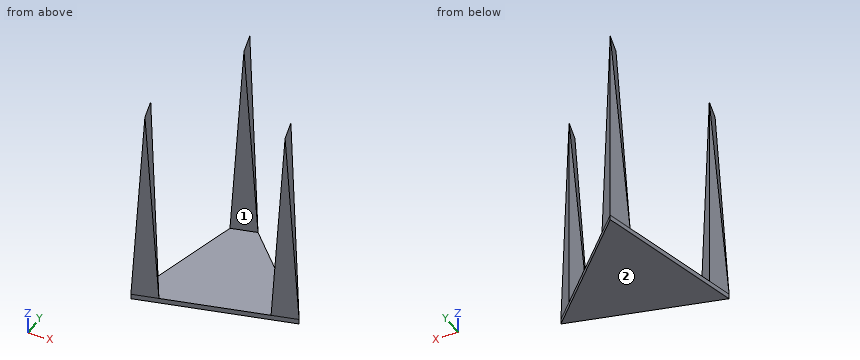
```python
from build123d import *

# Parameters (mm, degrees)
F1_DEPTH = 1
F3_DEPTH = 40
F5_DEPTH = 4.3311270189
F7_DEPTH = 25


with BuildPart() as f1:
    # F0 (on Top) → F1 (new body)
    with BuildSketch(Plane.XY):
        Polygon((2.8322214563, 24.2100603602), (-4.9323490894, -4.7677146448), (24.045425483, 2.9968575157), align=None)
    extrude(amount=F1_DEPTH)

    # F2 (on face) → F3 (join)
    with BuildSketch(Plane.XY.offset(1)):
        Polygon((-3.6382539984, 0.0619145227), (-4.9323490894, -4.7677146448), (-0.102719994, -3.4736192847), align=None)
        Polygon((6.3677554607, 20.6745265528), (2.8322214563, 24.2100603602), (1.5381263653, 19.3804311927), align=None)
        Polygon((19.2157963876, 1.7027621556), (24.045425483, 2.9968575157), (20.5098914785, 6.5323913231), align=None)
    extrude(amount=F3_DEPTH)

    # F4 (on face) → F5 (cut, through all)
    with BuildSketch(Plane(origin=(0.8615239687, -3.2152508648, 0), x_dir=(0.9659258191, 0.258819072, 0), z_dir=(0.258819072, -0.9659258191, 0))):
        Polygon((-5.9982588141, 41), (-5.9982588141, 1), (-3.4982588141, 41), align=None)
        Polygon((21.5017411859, 41), (24.0017411859, 1), (24.0017411859, 41), align=None)
        Polygon((-0.9982588141, 41), (-3.4982588141, 41), (-0.9982588141, 1), align=None)
        Polygon((19.0017411859, 41), (19.0017411859, 1), (21.5017411859, 41), align=None)
    extrude(amount=-F5_DEPTH, mode=Mode.SUBTRACT)

    # F6 (on face) → F7 (cut)
    with BuildSketch(Plane(origin=(-4.742073315, 17.6976565725, 0), x_dir=(0.9659258191, 0.258819072, 0), z_dir=(0.258819072, -0.9659258191, 0))):
        Polygon((6.5017411859, 41), (6.5017411859, 1), (9.0017411859, 41), align=None)
        Polygon((11.5017411859, 41), (9.0017411859, 41), (11.5017411859, 1), align=None)
    extrude(amount=-F7_DEPTH, mode=Mode.SUBTRACT)


solid = f1.part
```
Model file for the job. Use its own axes, mm. Face numbers are marked on the shaded views. A direction names the side the tool comes from. Coordinates: 2 decimals unless noted, no trailing zeros. Write each loop counter-clockwise with the first axis right and the second up, starting at its lowest first coordinate (ties: lowest second). Pieces come first, ordered by that corner, then holes. Notation, with made-up numbers: (21.5, 46) - (42.5, 46) arc R36 ccw to (42.5, 85) - close; hole circle Ø9 at (-22.5, -10.5). An arc over 180 degrees is marked (long way). Use a Markdown table: item, result. Add a question column.
Item 1: 3-axis set-ups, long thin cutter, end or side, ignore diameter. For the marked faces 1 and 2: which of +Z, -Z, +X, -X, +Y, -Y reach the whole face in a straight line?
Item 2: Band-saw the part on A-A, the plane z = 35.5. Write the cut outline in (x, y).
Item 3: Band-saw the part on C-C, the plane z = 20. Write the cut outline in (x, y), and give its area (3 significant figures).
Item 4: Drop flat-ended pins along their axis: pin 1 (1 mm diameter, centred on x = 0, z = 33.5, fed in from +Y); pin 2 (12 mm diameter, centred on y = 17, z = 22.5, fed in from +X); pin 3 (6 mm diameter, centred on x = 2.5, y = 4.5, fed in from +Z); pin 4 (10 mm diameter, centred on y = 4, z = 23.5, fed in from -X). Give the stop position or say it passes through.
Item 5: Band-saw the part on D-D, the plane y = 22.25. Write the cut outline in (x, z).
Item 6: Drill centre lines: line 1 along Z through (x, y) = (4, -2); line 2 along Y through (x, z) = (-1.75, 17) (3 decimals); line 3 along X through (y, z) = (5.75, 39). Where is each one in solid material? Low to high.
Item 7: Band-saw the part on B-B, the plane x = -1.75. Write the cut outline in (y, z) (3 decimals).
A:
| question | item | result |
|---|---|---|
| 1 | face 1 | +Z, +X, -Y |
| 1 | face 2 | -Z, +X, -X, +Y, -Y |
| 2 | outline | (-3.82, -0.6) - (-2.85, -4.21) - (-2.19, -4.03) - (-3.15, -0.42) - (-3.64, 0.06) - close; (2.65, 23.55) - (3.62, 19.94) - (4.28, 20.12) - (3.32, 23.72) - (2.83, 24.21) - close; (20.33, 5.87) - (21.3, 2.26) - (21.96, 2.44) - (21, 6.05) - (20.51, 6.53) - close |
| 3 | outline | (-4.32, -2.47) - (-3.79, -4.46) - (-1.25, -3.78) - (-1.78, -1.79) - (-3.64, 0.06) - close; (2.15, 21.67) - (2.69, 19.69) - (5.22, 20.37) - (4.69, 22.35) - (2.83, 24.21) - close; (19.83, 4) - (20.36, 2.01) - (22.9, 2.69) - (22.37, 4.68) - (20.51, 6.53) - close |
| 3 | area | 25.1 mm² |
| 4 | pin 1 | passes through |
| 4 | pin 2 | stops at x = 5.37 |
| 4 | pin 3 | stops at z = 1 |
| 4 | pin 4 | stops at x = -3.92 |
| 5 | outline | (2.31, 0) - (4.79, 0) - (4.79, 18.82) - (3.36, 41) - (2.31, 24.77) - close |
| 6 | line 1 | z = 0 to 1 |
| 6 | line 2 | y = -3.915 to -1.826 |
| 6 | line 3 | x = 20.59 to 20.85 |
| 7 | outline | (-3.915, 0) - (7.109, 0) - (7.109, 1) - (-1.826, 1) - (-1.826, 19.637) - (-3.915, 28.286) - close |
